Check sheet for the modelled part. Datum: model origin and axes. Units: mm. Face numbers are marked on the shaded views. A direction names the side the tool comes from. Round coordinates to 2 decimals unless told otherwise and drop trailing zeros. Order: outer loops, then holes, each group sorted by start corner. A loop starts at its lowest first (then second) coordinate and runs counter-clockwise, first axis right, second up.
from build123d import *

# Parameters (mm, degrees)
F0_W     = 55
F0_H     = 55
F1_DEPTH = 3
F2_W     = 55
F2_H     = 55
F2_W_2   = 51
F2_H_2   = 51
F3_DEPTH = 10
F4_R     = 2.8
F5_DEPTH = 5
F6_W     = 4
F6_H     = 4
F7_DEPTH = 25
F9_DEPTH = 2.4
F10_R    = 1.99999


# Not quite as in the source:
# - a fillet or chamfer is up to 0.001 mm smaller than in the source, because OpenCascade refuses the exact size


with BuildPart() as f1:
    # F0 (on Top) → F1 (new body)
    with BuildSketch(Plane.XY):
        Rectangle(F0_W, F0_H)
    extrude(amount=F1_DEPTH)

    # F2 (on face) → F3 (join)
    with BuildSketch(Plane.XY.offset(3)):
        Rectangle(F2_W, F2_H)
        Rectangle(F2_W_2, F2_H_2, mode=Mode.SUBTRACT)
    extrude(amount=F3_DEPTH)

    # F4 (on face) → F5 (join)
    with BuildSketch(Plane.XY.offset(3)):
        with Locations((-20.3, -20.3)):
            Circle(F4_R)
        with Locations((20.3, 20.3)):
            Circle(F4_R)
    extrude(amount=F5_DEPTH)

    # F6 (on face) → F7 (cut)
    with BuildSketch(Plane.XY.offset(13)):
        with Locations((-25.5, 25.5)):
            Rectangle(F6_W, F6_H)
        with Locations((25.5, -25.5)):
            Rectangle(F6_W, F6_H)
    extrude(amount=-F7_DEPTH, mode=Mode.SUBTRACT)

    # F8 (on face) → F9 (cut)
    with BuildSketch(Plane.XY.offset(3)):
        Polygon((-23.5, 25.5), (-25.5, 23.5), (23.5, -25.5), (25.5, -23.5), align=None)
    extrude(amount=-F9_DEPTH, mode=Mode.SUBTRACT)

    # F10 (radius 2 in the source; OpenCascade refuses exactly that, so slightly less here)
    f10_edges = [f1.edges().sort_by_distance(p)[0] for p in [
        (-26.5, 23.5, 13),
        (23.5, -26.5, 13),
        (26.5, -23.5, 13),
        (-23.5, 26.5, 13),
        (-27.5, 23.5, 6.5),
        (-23.5, 27.5, 6.5),
        (23.5, -27.5, 6.5),
        (27.5, -23.5, 6.5),
        (-27.5, -27.5, 6.5),
        (27.5, 27.5, 6.5),
    ]]
    fillet(f10_edges, radius=F10_R)


solid = f1.part
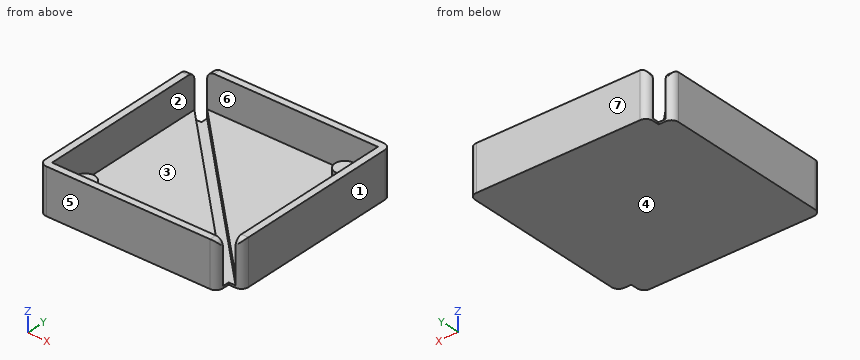
1) Draft check along Y on the marked faces 4, 5, 6 and 7. Enter one of: pulls with the +Y half, pulls with the -Y half, needs draft (parallel to the pull), parting line crosses it, or undercut.
2) Sectioned sample at B-B on y = 20.3. Record the cut outline in (x, z).
3) Scan lines: line 1 (X direction, y = -1.5, z = 9.5); line 2 (Y direction, x = -20.5, z = 7.75). Record each from-to range of solid material in increasing order.
4) Set-up check for the marked faces 1, 2 and 3: record each of +Z, -Z, +X, -X, +Y, -Y from which the full face is reachable in a straight line by a thin tool's end or side.
5) Sectioned sample at C-C on x = 10. Record the cut outline in (y, z).
6) Sectioned sample at D-D on y = -14. Record the cut outline in (x, z), and give its area (3 significant figures).
7) Gauge pin test, flat ends, axial feed: pin 1 (4.5 mm diameter, centred on x = 20, y = 21.5, fed in from +Z); pin 2 (0.6 mm diameter, centred on y = 24.5, z = 7.5, fed in from -X); pin 3 (0.6 mm diameter, centred on x = -24.5, z = 4.5, fed in from +Y). Record the tip position at first contact, or that the pin passes through.
Values found:
1. face 4: needs draft
1. face 5: pulls with the -Y half
1. face 6: undercut
1. face 7: pulls with the +Y half
2. outline: (-27.5, 0) - (27.5, 0) - (27.5, 13) - (25.5, 13) - (25.5, 3) - (23.1, 3) - (23.1, 8) - (17.5, 8) - (17.5, 3) - (-18.3, 3) - (-18.3, 0.6) - (-22.3, 0.6) - (-22.3, 3) - (-25.5, 3) - (-25.5, 13) - (-27.5, 13) - close
3. line 1: x = -27.5 to -25.5, 25.5 to 27.5
3. line 2: y = -27.5 to -25.5, -23.09 to -17.51, 25.5 to 27.5
4. face 1: +Z, -Z, +X, +Y, -Y
4. face 2: +Z, +Y
4. face 3: +Z
5. outline: (-27.5, 0) - (27.5, 0) - (27.5, 13) - (25.5, 13) - (25.5, 3) - (-8, 3) - (-8, 0.6) - (-12, 0.6) - (-12, 3) - (-25.5, 3) - (-25.5, 13) - (-27.5, 13) - close
6. outline: (-27.5, 0) - (27.5, 0) - (27.5, 13) - (25.5, 13) - (25.5, 3) - (16, 3) - (16, 0.6) - (12, 0.6) - (12, 3) - (-25.5, 3) - (-25.5, 13) - (-27.5, 13) - close
6. area: 195 mm2
7. pin 1: stops at z = 8
7. pin 2: stops at x = 25.5
7. pin 3: stops at y = -25.5
